```python
from build123d import *

# Parameters (mm, degrees)
BOSS_EXTRUDE1_DEPTH = 49
BOSS_EXTRUDE3_DEPTH = 10.5
CHAMFER1_SIZE       = 3
SKETCH4_R           = 2.1
CUT_EXTRUDE1_DEPTH  = 23
SKETCH5_W           = 8
SKETCH5_H           = 10
CUT_EXTRUDE2_DEPTH  = 21
BOSS_EXTRUDE5_DEPTH = 1.5
SKETCH6_W           = 12
SKETCH6_H           = 20
CUT_EXTRUDE3_DEPTH  = 5
FILLET1_R           = 2


with BuildPart() as part:
    # Sketch1 → Boss-Extrude1 (new body, symmetric)
    with BuildSketch(Plane.XY):
        Polygon((-29.5, 0), (-17.5, 0), (-17.5, -20), (17.5, -20), (17.5, 0), (29.5, 0), (29.5, -2), (19.5, -2), (19.5, -22), (-19.5, -22), (-19.5, -2), (-29.5, -2), align=None)
    extrude(amount=BOSS_EXTRUDE1_DEPTH, both=True)

    # Sketch3 → Boss-Extrude3 (add, symmetric)
    with BuildSketch(Plane(origin=(0, 0, 0), x_dir=(0, 0, -1), z_dir=(1, 0, 0))):
        Polygon((-49, -22), (-63, -22), (-63, -6), (-61, -6), (-61, -20), (-49, -20), align=None)
    extrude(amount=BOSS_EXTRUDE3_DEPTH, both=True)

    # Chamfer1
    chamfer1_edges = [part.edges().sort_by_distance(p)[0] for p in [
        (19.5, -2, 0),
        (-19.5, -2, 0),
    ]]
    chamfer(chamfer1_edges, length=CHAMFER1_SIZE)

    # Sketch4 → Cut-Extrude1 (cut, through all)
    with BuildSketch(Plane(origin=(0, 0, 0), x_dir=(1, 0, 0), z_dir=(0, 1, 0))):
        with Locations((-23.5, 0)):
            Circle(SKETCH4_R)
        with Locations((23.5, 0)):
            Circle(SKETCH4_R)
    extrude(amount=-CUT_EXTRUDE1_DEPTH, mode=Mode.SUBTRACT)

    # Sketch5 → Cut-Extrude2 (cut, through all)
    with BuildSketch(Plane.XZ.offset(2)):
        with Locations((23.5, 0)):
            Rectangle(SKETCH5_W, SKETCH5_H)
        with Locations((-23.5, 0)):
            Rectangle(SKETCH5_W, SKETCH5_H)
    extrude(amount=CUT_EXTRUDE2_DEPTH, mode=Mode.SUBTRACT)

    # Sketch2 → Boss-Extrude5 (add)
    with BuildSketch(Plane(origin=(0, 0, -49), x_dir=(-1, 0, 0), z_dir=(0, 0, -1))):
        Polygon((-17.5, 0), (17.5, 0), (29.5, 0), (29.5, -2), (22.5, -2), (19.5, -5), (19.5, -22), (-19.5, -22), (-19.5, -5), (-22.5, -2), (-29.5, -2), (-29.5, 0), align=None)
    extrude(amount=BOSS_EXTRUDE5_DEPTH)

    # Sketch6 → Cut-Extrude3 (cut)
    with BuildSketch(Plane(origin=(0, 0, 0), x_dir=(1, 0, 0), z_dir=(0, 1, 0))):
        with Locations((-23.5, -39)):
            Rectangle(SKETCH6_W, SKETCH6_H)
        with Locations((23.5, -39)):
            Rectangle(SKETCH6_W, SKETCH6_H)
        with Locations((23.5, 40.5)):
            Rectangle(SKETCH6_W, SKETCH6_H)
        with Locations((-23.5, 40.5)):
            Rectangle(SKETCH6_W, SKETCH6_H)
    extrude(amount=-CUT_EXTRUDE3_DEPTH, mode=Mode.SUBTRACT)

    # Fillet1
    fillet1_edges = [part.edges().sort_by_distance(p)[0] for p in [
        (-29.5, -1, -30.5),
        (29.5, -1, -30.5),
        (29.5, -1, 29),
        (-29.5, -1, 29),
        (-10.5, -6, 62),
        (10.5, -6, 62),
    ]]
    fillet(fillet1_edges, radius=FILLET1_R)


solid = part.part
```
Source: CAD feature listing. Evaluate the final solid. Frame: model axes, mm. A direction names the side the tool comes from. Round coordinates to 2 decimals unless told otherwise and drop trailing zeros. Write each loop counter-clockwise with the first axis right and the second up, starting at its lowest first coordinate (ties: lowest second). Pieces come first, ordered by that corner, then holes. Notation, with made-up numbers: M 34,-1.75 L 63,-1.75 A22 cw 63,20.25 Z; hole C 36,-8 d6. An arc over 180 degrees is marked long. Answer as a JSON object with one key per item and string values. Group by question number.
(1) Section query D-D on z = 21. Output: boundary loops of the cut face in (x, y).
(2) Section query A-A on z = 0. Output: boundary loops of the cut face in (x, y).
(3) Section query B-B on y = -12.5. Output: boundary loops of the cut face in (x, z), then the cut area to 4 significant figures.
(4) Section query C-C on x = -7. Output: boundary loops of the cut face in (y, z), then the cut area to 3 significant figures.
(5) Mould query, pull axis X, two halves, no side actions, for faces 1 (the flat face through (0, -13, 61)), 2 (the flat face through (-17.5, -10, 1)), 3 (the cylindrical face through (-28.93, -1.01, 28.4)). Classes: +X half, -X half, draft (parallel to the pull), parting line (faces both ways), or undercut.
(6) Reachability of faces 4 (the flat face through (21, -2, 29)), 5 (the flat face through (0, -20, 7)), 6 (the flat face through (-10.5, -17.6, 61.2)), 7 (the flat face through (10.5, -17.6, 61.2)), 8 (the flat face through (21, -2, -30.5)) from +Z, -Z, +X, -X, +Y, -Y: full face, straight path, thin tool, end or side. Return the list, or none.
(7) First-contact query: pin 1 (1.2 mm diameter, centred on y = -1.5, z = -49.5, fed in from -X); pin 2 (1.6 mm diameter, centred on x = -18.5, z = 44, fed in from +Y); pin 3 (4 mm diameter, centred on x = 11, z = 22, fed in from +Y). Flat tips, straight axial feed; report the tip coordinate or a pass-through.
(8) Ray query, line 1 (X direction, y = -0.6, z = 0); line 2 (X direction, y = -14.25, z = -29); line 3 (Z direction, x = 23.5, y = -1.1). Return the intervals inside material, ascending. Write a range as [from, to].
Computed values:
{
 "1": {"outline": "M -29.5,-2 L -22.5,-2 L -19.5,-5 L -19.5,-22 L 19.5,-22 L 19.5,-5 L 22.5,-2 L 29.5,-2 L 29.5,0 L 17.5,0 L 17.5,-20 L -17.5,-20 L -17.5,0 L -29.5,0 Z"},
 "2": {"outline": "M -29.5,-2 L -25.6,-2 L -25.6,0 L -29.5,0 Z; M -21.4,-2 L -19.5,-2 L -19.5,-22 L 19.5,-22 L 19.5,-2 L 21.4,-2 L 21.4,0 L 17.5,0 L 17.5,-20 L -17.5,-20 L -17.5,0 L -21.4,0 Z; M 25.6,-2 L 29.5,-2 L 29.5,0 L 25.6,0 Z"},
 "3": {"outline": "M -19.5,-50.5 L 19.5,-50.5 L 19.5,49 L 17.5,49 L 17.5,-49 L -17.5,-49 L -17.5,49 L -19.5,49 Z; M -10.5,61 L 10.5,61 L 10.5,63 L -10.5,63 Z", "area": "492.5 mm^2"},
 "4": {"outline": "M -22,-50.5 L 0,-50.5 L 0,-49 L -20,-49 L -20,61 L -6,61 L -6,63 L -22,63 Z", "area": "285 mm^2"},
 "5": {"face 1": "draft", "face 2": "undercut", "face 3": "-X half"},
 "6": {"face 4": "+Z, +X, -X, +Y", "face 5": "+Y", "face 6": "+Z, -X, +Y, -Y", "face 7": "+Z, +X, +Y, -Y", "face 8": "-Z, +X, -X, +Y"},
 "7": {"pin 1": "x = -17.5", "pin 2": "y = -5", "pin 3": "y = -20"},
 "8": {"line 1": "[-29.5, -25.6], [-21.4, -17.5], [17.5, 21.4], [25.6, 29.5]", "line 2": "[-19.5, -17.5], [17.5, 19.5]", "line 3": "[-30.5, -2.1], [2.1, 29]"}
}
